Autodesk Inventor part; units mm, degrees
ref_plane "YZ Plane" through (0, 0, 0) normal (1, 0, 0) x (0, 1, 0)
ref_plane "XZ Plane" through (0, 0, 0) normal (0, 1, 0) x (-1, 0, 0)
ref_plane "XY Plane" through (0, 0, 0) normal (0, 0, 1) x (1, 0, 0)
ref_plane "Arbeitsebene1" through (-0.0002, 0, 0) normal (0, 0, 1) x (1, 0, 0)
sketch "Skizze1" plane through (-0.0002, 0, 0) normal (0, 0, 1) x (1, 0, 0)
  circle A0 centre (13.85, 6.86) radius 1.5
  circle A1 centre (0.85, 31.86) radius 1.5
  circle A2 centre (13.85, 31.86) radius 1.5
  circle A3 centre (0.85, 6.86) radius 1.5
  circle A4 centre (5.0933, 19.36) radius 5.5
  line L0 (-3.07, 5.49) -> (-3.07, 33.23)
  line L1 (-3.07, 5.49) -> (-16.87, 5.49)
  line L2 (-16.87, 13.31) -> (-16.87, 5.49)
  line L3 (-16.8476, 13.31) -> (-16.87, 13.31)
  line L4 (-16.8476, 25.41) -> (-16.8476, 13.31)
  line L5 (-16.87, 25.41) -> (-16.8476, 25.41)
  line L6 (-16.87, 33.23) -> (-16.87, 25.41)
  line L7 (-3.07, 33.23) -> (-16.87, 33.23)
  line L8 (-16.87, 40.13) -> (-16.87, 44.21)
  line L9 (-20.77, 36.23) -> (-16.87, 40.13)
  line L10 (-24.85, 36.23) -> (-20.77, 36.23)
  line L11 (-24.85, 2.49) -> (-24.85, 36.23)
  line L12 (-20.77, 2.49) -> (-24.85, 2.49)
  line L13 (-16.87, -1.41) -> (-20.77, 2.49)
  line L14 (-16.87, -1.41) -> (-16.87, -5.49)
  line L15 (-16.87, -5.49) -> (16.87, -5.49)
  line L16 (16.87, -5.49) -> (16.87, -1.41)
  line L17 (20.77, 2.49) -> (16.87, -1.41)
  line L18 (24.85, 2.49) -> (20.77, 2.49)
  line L19 (24.85, 36.23) -> (24.85, 2.49)
  line L20 (20.77, 36.23) -> (24.85, 36.23)
  line L21 (16.87, 40.13) -> (20.77, 36.23)
  line L22 (16.87, 44.21) -> (16.87, 40.13)
  line L23 (-16.87, 44.21) -> (16.87, 44.21)
  line L24 (16.97, 36.33) -> (16.97, 2.39)
  line L25 (-16.97, 36.33) -> (16.97, 36.33) construction
  line L26 (-16.97, 2.39) -> (-16.97, 36.33)
  line L27 (16.97, 2.39) -> (-16.97, 2.39) construction
  line L28 (16.97, 2.39) -> (-16.97, 2.39)
  line L29 (16.47, 35.83) -> (16.47, 2.89)
  line L30 (16.47, 2.89) -> (-16.47, 2.89)
  line L31 (-16.47, 2.89) -> (-16.47, 35.83)
  line L32 (-16.47, 35.83) -> (16.47, 35.83)
  line L33 (-2.57, 35.83) -> (-2.57, 2.89)
  circle A5 centre (5.0933, 19.36) radius 3.505
  circle A6 centre (5.0933, 19.36) radius 3
  point P0 (0.0002, 0)
extrude "Extrusion1" add sketch "Skizze1" along normal blind 5 contours A4 | L33 L32 L29 L30 | A5
sketch "Skizze5" plane through (16.4698, 2.89, 0) normal (1, 0, 0) x (0, 0, -1)
  line L0 (-23, 19.975) -> (-13.08, 19.975)
  line L1 (-23, 12.965) -> (-13.08, 12.965)
  circle A0 centre (-2.5, 20.5313) radius 1.4
  circle A1 centre (-2.5, 12.3138) radius 1.4
  line L2 (0, 0) -> (0, 32.94)
  line L3 (0, 32.94) -> (-5, 32.94)
  line L4 (-5, 0) -> (-5, 32.94)
  line L5 (0, 0) -> (-5, 0)
  line L6 (-5, 13.47) -> (-5, 19.47)
  line L7 (0, 13.47) -> (0, 19.47)
  line L8 (-5, 32.94) -> (-5, 0)
  line L9 (-5, 0) -> (-5, 32.94)
  line L10 (-5, 2.47) -> (-5, 5.47)
  line L11 (-5, 27.47) -> (-5, 30.47)
  line L12 (-5, 27.47) -> (-5, 30.47)
  line L13 (-5, 2.47) -> (-5, 5.47)
  line L14 (-5, 13.47) -> (-5, 19.47)
  line L15 (-5, 19.47) -> (0, 19.47)
  line L16 (-5, 13.47) -> (0, 13.47)
  point P0 (0, -2.89)
  dimension "d19" = 2.8
  dimension "d20" = 2.8
hole "Bohrung2" at (16.4698, 23.4213, 2.5) at (16.4698, 15.2038, 2.5) direction (-1, 0, 0) diameter 2.8 depth 30 counterbore diameter 6.5 counterbore depth 3
properties part number "30_Cube_Z_Focus_NEMA8_captive_micrometerscrewbase_v0"
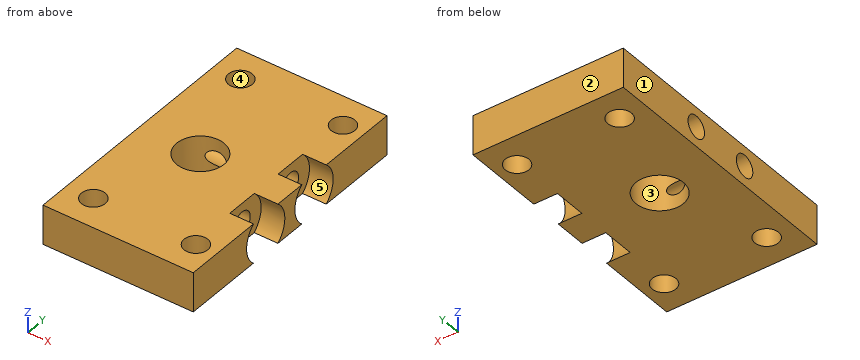
The model under review builds one solid part; all positions refer to its coordinate system, in mm. Face numbers are marked on the shaded views. A direction names the side the tool comes from. Round coordinates to 2 decimals unless told otherwise and drop trailing zeros. Order: outer loops, then holes, each group sorted by start corner. A loop starts at its lowest first (then second) coordinate and runs counter-clockwise, first axis right, second up.
Item 1: Machinability: for the marked faces 4 and 5, which of the approach directions +Z, -Z, +X, -X, +Y, -Y give a long, thin tool a straight path to every point of the face, cutting with its end or side? Answer none if there is none.
Working result:
face 4: +Z, -Z
face 5: +X
Item 2: Add section B-B, the plane z = 2.5. State the section outline as (x, y) points, and give its area (3 significant figures).
Working result:
outline: (-2.57, 2.89) - (16.47, 2.89) - (16.47, 11.95) - (13.47, 11.95) - (13.47, 13.8) - (-2.57, 13.8) - close; (-2.57, 16.6) - (3.91, 16.6) arc R3 cw to (3.71, 22.02) - (-2.57, 22.02) - close; (-2.57, 24.82) - (13.47, 24.82) - (13.47, 26.67) - (16.47, 26.67) - (16.47, 35.83) - (-2.57, 35.83) - close; (6.28, 16.6) - (13.47, 16.6) - (13.47, 18.45) - (16.47, 18.45) - (16.47, 20.17) - (13.47, 20.17) - (13.47, 22.02) - (6.48, 22.02) arc R3 cw to start; hole circle Ø3 at (0.85, 6.86); hole circle Ø3 at (0.85, 31.86); hole circle Ø3 at (13.85, 6.86); hole circle Ø3 at (13.85, 31.86)
area: 443 mm2
Item 3: For pin 1 (3 mm diameter, centred on y = 15.2, z = 2.5, fed in from +X); pin 2 (2.5 mm diameter, centred on x = 0.85, y = 6.86, fed in from +Z), all flat-tipped, find the tip position at first contact; note any pin that passes through.
Working result:
pin 1: stops at x = 13.47
pin 2: passes through
Item 4: Draft analysis for pull direction X (two halves, no side actions). For the marked faces 1, 2 and 3, state which applies: released by +X, released by -X, zero draft, split by the parting line, or undercut.
Working result:
face 1: released by -X
face 2: zero draft
face 3: undercut
Item 5: Add section A-A, the plane y = 19.36. State the section outline as (x, z) points.
Working result:
outline: (-2.57, 0) - (2.09, 0) - (2.09, 5) - (-2.57, 5) - close; (8.09, 0) - (16.47, 0) - (16.47, 5) - (8.09, 5) - close
Item 6: To check wall thickness, follow probe 1 along Y at (x, z) = (9, 2.6); probe 2 along Y at (x, z) = (15.5, 0.65); probe 3 along Y at (x, z) = (14.25, 2.9). State the ranges of each line that lie inside material, in increasing order.
Working result:
probe 1: y = 2.89 to 13.81, 16.6 to 22.02, 24.82 to 35.83
probe 2: y = 2.89 to 12.53, 17.88 to 20.75, 26.09 to 35.83
probe 3: y = 2.89 to 5.41, 8.31 to 11.98, 18.43 to 20.2, 26.65 to 30.41, 33.31 to 35.83
Item 7: Add section D-D, the plane y = 6.86. State the section outline as (x, z) points.
Working result:
outline: (-2.57, 0) - (-0.65, 0) - (-0.65, 5) - (-2.57, 5) - close; (2.35, 0) - (12.35, 0) - (12.35, 5) - (2.35, 5) - close; (15.35, 0) - (16.47, 0) - (16.47, 5) - (15.35, 5) - close
Item 8: Add section C-C, the plane x = 3.25. State the section outline as (y, z) points.
Working result:
outline: (2.89, 0) - (16.99, 0) - (16.99, 5) - (2.89, 5) - close; (21.73, 0) - (35.83, 0) - (35.83, 5) - (21.73, 5) - close; hole circle Ø2.8 at (15.2, 2.5); hole circle Ø2.8 at (23.42, 2.5)
